from build123d import *

# Parameters (mm, degrees)
F0_R     = 3.175
F0_W     = 7.62
F0_H     = 7.62
F0_R_2   = 1.27
F0_W_2   = 2.54
F0_H_2   = 13.462
F1_DEPTH = 2.54
F2_DEPTH = 3.81
F3_DEPTH = 6.35
F4_DEPTH = 22.86
F5_R     = 5.08
F5_R_2   = 5.3975
F5_R_3   = 3.175
F5_R_4   = 3.81
F6_DEPTH = 1.905
F8_DEPTH = 1.905
F9_START = -68.453
F9_DEPTH = 1.905


with BuildPart() as f1:
    # F0 (on Top) → F1 (new body)
    with BuildSketch(Plane.XY):
        Polygon((-32.385, 65.278), (-32.385, 57.15), (-16.51, 57.15), (-16.51, 65.278), (1.27, 65.278), (1.27, 67.183), (-18.415, 67.183), (-18.415, 59.055), (-30.48, 59.055), (-30.48, 67.183), (-40.005, 67.183), (-40.005, 65.278), align=None)
        Polygon((-16.51, 57.15), (-32.385, 57.15), (-32.385, 65.278), (-40.005, 65.278), (-43.18, 65.278), (-43.18, 80.645), (-67.945, 80.645), (-67.945, 67.183), (-67.945, 57.15), (-106.68, 57.15), (-106.68, 49.53), (-114.3, 49.53), (-114.3, 6.35), (-106.68, 6.35), (-106.68, -1.27), (1.27, -1.27), (1.27, 65.278), (-16.51, 65.278), align=None)
        with Locations((-5.08, 3.81)):
            Circle(F0_R, mode=Mode.SUBTRACT)
        with Locations((-20.32, 52.07)):
            Circle(F0_R, mode=Mode.SUBTRACT)
        with Locations((-110.49, 53.34)):
            Rectangle(F0_W, F0_H)
        with Locations((-110.49, 2.54)):
            Rectangle(F0_W, F0_H)
        Polygon((-67.945, 80.645), (-43.18, 80.645), (-40.005, 80.645), (-40.005, 87.63), (-70.485, 87.63), (-70.485, 80.645), align=None)
        with Locations((-68.58, 83.185)):
            Circle(F0_R_2, mode=Mode.SUBTRACT)
        with Locations((-41.91, 83.185)):
            Circle(F0_R_2, mode=Mode.SUBTRACT)
        with Locations((-68.58, 83.185)):
            Circle(F0_R_2)
        with Locations((-41.91, 83.185)):
            Circle(F0_R_2)
        with Locations((-20.32, 52.07)):
            Circle(F0_R)
        with Locations((-20.32, 52.07)):
            Circle(F0_R_2, mode=Mode.SUBTRACT)
        with Locations((-20.32, 52.07)):
            Circle(F0_R_2)
        with Locations((-5.08, 3.81)):
            Circle(F0_R)
        with Locations((-5.08, 3.81)):
            Circle(F0_R_2, mode=Mode.SUBTRACT)
        with Locations((-5.08, 3.81)):
            Circle(F0_R_2)
        Polygon((1.27, -3.175), (1.27, -1.27), (-106.68, -1.27), (-114.3, -1.27), (-114.3, 6.35), (-114.3, 49.53), (-114.3, 57.15), (-106.68, 57.15), (-67.945, 57.15), (-67.945, 67.183), (-70.485, 67.183), (-70.485, 59.055), (-116.205, 59.055), (-116.205, -3.175), align=None)
        Polygon((1.27, 67.183), (1.27, 65.278), (1.27, -1.27), (1.27, -3.175), (3.175, -3.175), (3.175, 67.183), align=None)
        with Locations((-69.215, 73.914)):
            Rectangle(F0_W_2, F0_H_2)
        Polygon((-43.18, 65.278), (-40.005, 65.278), (-40.005, 67.183), (-40.005, 80.645), (-43.18, 80.645), align=None)
    extrude(amount=-F1_DEPTH)

    # F0 (on Top) → F2 (join)
    with BuildSketch(Plane.XY):
        Polygon((-67.945, 80.645), (-43.18, 80.645), (-40.005, 80.645), (-40.005, 87.63), (-70.485, 87.63), (-70.485, 80.645), align=None)
        with Locations((-68.58, 83.185)):
            Circle(F0_R_2, mode=Mode.SUBTRACT)
        with Locations((-41.91, 83.185)):
            Circle(F0_R_2, mode=Mode.SUBTRACT)
        with Locations((-110.49, 53.34)):
            Rectangle(F0_W, F0_H)
        with Locations((-110.49, 2.54)):
            Rectangle(F0_W, F0_H)
        with Locations((-20.32, 52.07)):
            Circle(F0_R)
        with Locations((-20.32, 52.07)):
            Circle(F0_R_2, mode=Mode.SUBTRACT)
        with Locations((-5.08, 3.81)):
            Circle(F0_R)
        with Locations((-5.08, 3.81)):
            Circle(F0_R_2, mode=Mode.SUBTRACT)
        with Locations((-68.58, 83.185)):
            Circle(F0_R_2)
        with Locations((-41.91, 83.185)):
            Circle(F0_R_2)
        with Locations((-20.32, 52.07)):
            Circle(F0_R_2)
        with Locations((-5.08, 3.81)):
            Circle(F0_R_2)
    extrude(amount=F2_DEPTH)

    # F0 (on Top) → F3 (join)
    with BuildSketch(Plane.XY):
        with Locations((-68.58, 83.185)):
            Circle(F0_R_2)
        with Locations((-41.91, 83.185)):
            Circle(F0_R_2)
        with Locations((-20.32, 52.07)):
            Circle(F0_R_2)
        with Locations((-5.08, 3.81)):
            Circle(F0_R_2)
        Polygon((1.27, -3.175), (1.27, -1.27), (-106.68, -1.27), (-114.3, -1.27), (-114.3, 6.35), (-114.3, 49.53), (-114.3, 57.15), (-106.68, 57.15), (-67.945, 57.15), (-67.945, 67.183), (-70.485, 67.183), (-70.485, 59.055), (-116.205, 59.055), (-116.205, -3.175), align=None)
        Polygon((-32.385, 65.278), (-32.385, 57.15), (-16.51, 57.15), (-16.51, 65.278), (1.27, 65.278), (1.27, 67.183), (-18.415, 67.183), (-18.415, 59.055), (-30.48, 59.055), (-30.48, 67.183), (-40.005, 67.183), (-40.005, 65.278), align=None)
    extrude(amount=F3_DEPTH)

    # F0 (on Top) → F4 (join)
    with BuildSketch(Plane.XY):
        Polygon((1.27, 67.183), (1.27, 65.278), (1.27, -1.27), (1.27, -3.175), (3.175, -3.175), (3.175, 67.183), align=None)
    extrude(amount=F4_DEPTH)

    # F5 (on face) → F6 (cut, through all)
    with BuildSketch(Plane.YZ.offset(3.175)):
        with Locations((15.875, 12.319)):
            Circle(F5_R)
        with Locations((32.512, 11.43)):
            Circle(F5_R_2)
        with Locations((46.99, 12.319)):
            Circle(F5_R_3)
        with Locations((59.182, 10.414)):
            Circle(F5_R_4)
    extrude(amount=-F6_DEPTH, mode=Mode.SUBTRACT)

    # F7 (on face) → F8 (join, through all)
    with BuildSketch(Plane(origin=(0, 67.183, 0), x_dir=(-1, 0, 0), z_dir=(0, 1, 0))):
        Polygon((6.4287394361, 6.35), (-1.27, 22.86), (-1.27, 6.35), align=None)
    extrude(amount=-F8_DEPTH)

    # F7 (on face) → F9 (join)
    with BuildSketch(Plane(origin=(0, 67.183, 0), x_dir=(-1, 0, 0), z_dir=(0, 1, 0)).offset(F9_START)):
        Polygon((6.4287394361, 6.35), (-1.27, 22.86), (-1.27, 6.35), align=None)
    extrude(amount=-F9_DEPTH)


solid = f1.part
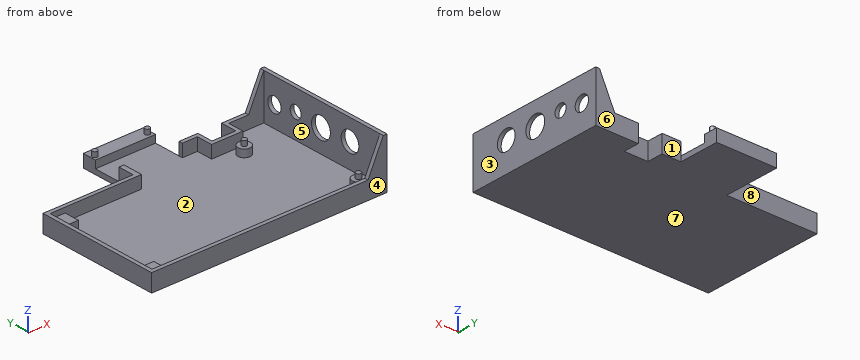
Source: CAD feature listing. Evaluate the final solid. Frame: model axes, mm. Face numbers are marked on the shaded views. A direction names the side the tool comes from. Round coordinates to 2 decimals unless told otherwise and drop trailing zeros. Loops run counter-clockwise (first coordinate to the right, second up) from the corner with the lowest first, then second, coordinate; pieces in that order, holes last. Notation, with made-up numbers: (69.5, 16.5) -> (93.5, 16.5) arc R29 cw to (93.5, 41.5) -> close; hole circle Ø2 at (40, 33.5). An arc over 180 degrees is marked (long way). Answer as a JSON object with one key per item and string values. Group by question number.
Q1. Section query C-C (y = 3.81). Output: boundary loops of the cut face in (x, z) (3 decimals), plus the area to 3 significant figures.
Q2. Section query A-A (x = -10). Output: boundary loops of the cut face in (y, z) (3 decimals).
Q3. Mould query, pull axis Y, two halves, no side actions, for the marked faces 1, 2 and 3. Classes: pulls with the +Y half, pulls with the -Y half, needs draft (parallel to the pull), parting line crosses it, or undercut.
Q4. Section query B-B (y = 45.5). Output: boundary loops of the cut face in (x, z) (3 decimals).
Q5. Ray query, line 1 (X direction, y = 59, z = 1.5) (3 decimals); line 2 (X direction, y = 41.5, z = 4.25) (3 decimals); line 3 (Y direction, x = -88.5, z = 4) (3 decimals). Return the intervals inside material, ascending. Write a range as from..to.
Q6. Section query D-D (x = -41.91). Output: boundary loops of the cut face in (y, z) (3 decimals), plus the area to 3 significant figures.
Q7. Contact query for flat-ended pins moving along their axis: P1, Ø8, axis at x = -20.5, y = 64.5, coming from the +Z side; P2, Ø21, axis at x = -88, y = 35, coming from the +Z side; P3, Ø0.6, axis at y = 66, z = 4.5, coming from the -X side (3 decimals). Output: stop coordinate, or through.
Q8. Access query for the marked faces 4, 5, 6, 7 and 8. Directions: +Z, -Z, +X, -X, +Y, -Y. A direction counts if a zero-diameter tool reaches every point of the face in a straight line with its end or side. Return the directions, or none.
Completed:
{
 "1": {"outline": "(-116.205, -2.54) -> (3.175, -2.54) -> (3.175, 22.86) -> (1.27, 22.86) -> (1.27, 0) -> (-1.905, 0) -> (-1.905, 3.81) -> (-3.81, 3.81) -> (-3.81, 6.35) -> (-6.35, 6.35) -> (-6.35, 3.81) -> (-8.255, 3.81) -> (-8.255, 0) -> (-106.68, 0) -> (-106.68, 3.81) -> (-114.3, 3.81) -> (-114.3, 6.35) -> (-116.205, 6.35) -> close", "area": "419 mm²"},
 "2": {"outline": "(-3.175, -2.54) -> (67.183, -2.54) -> (67.183, 6.35) -> (65.278, 6.35) -> (65.278, 0) -> (-1.27, 0) -> (-1.27, 6.35) -> (-3.175, 6.35) -> close"},
 "3": {"face 1": "pulls with the +Y half", "face 2": "undercut", "face 3": "needs draft"},
 "4": {"outline": "(-116.205, -2.54) -> (3.175, -2.54) -> (3.175, 9.515) -> (1.27, 9.515) -> (1.27, 0) -> (-114.3, 0) -> (-114.3, 6.35) -> (-116.205, 6.35) -> close; (1.27, 15.123) -> (3.175, 15.123) -> (3.175, 22.86) -> (1.27, 22.86) -> close"},
 "5": {"line 1": "-116.205..-67.945, -32.385..-16.51, 1.27..3.175", "line 2": "-116.205..-114.3, 1.27..3.175", "line 3": "-3.175..-1.27, 57.15..59.055"},
 "6": {"outline": "(-3.175, -2.54) -> (87.63, -2.54) -> (87.63, 3.81) -> (84.455, 3.81) -> (84.455, 6.35) -> (81.915, 6.35) -> (81.915, 3.81) -> (80.645, 3.81) -> (80.645, 0) -> (-1.27, 0) -> (-1.27, 6.35) -> (-3.175, 6.35) -> close", "area": "276 mm²"},
 "7": {"P1": "z = 6.35", "P2": "z = 0", "P3": "x = -70.485"},
 "8": {"face 4": "+Z, -Z, +X, -X, -Y", "face 5": "+Z", "face 6": "+Z, -Z, +X, +Y", "face 7": "-Z, +X, -X, +Y, -Y", "face 8": "+Z, -Z, -X, +Y"}
}
